Autodesk Inventor part; units mm, degrees
ref_plane "YZ Plane" through (0, 0, 0) normal (1, 0, 0) x (0, 1, 0)
ref_plane "XZ Plane" through (0, 0, 0) normal (0, 1, 0) x (-1, 0, 0)
ref_plane "XY Plane" through (0, 0, 0) normal (0, 0, 1) x (1, 0, 0)
sketch "Sketch1" plane through (0, 0, 0) normal (0, 0, 1) x (1, 0, 0)
  line L0 (0, 0) -> (609.6, 0)
  line L1 (609.6, 0) -> (609.6, 25.4)
  line L2 (609.6, 25.4) -> (0, 25.4)
  line L3 (0, 25.4) -> (0, 0)
  dimension "d0" = 25.4
  dimension "d1" = 609.6
extrude "Extrusion1" add sketch "Sketch1" along normal blind 25.4
shell "Shell1" thickness 1.5875 removed faces 2 at (0, 16.9333, 8.4667) at (609.6, 8.4667, 8.4667)
sketch "Sketch2" plane through (0, 0, 25.4) normal (0, 0, 1) x (1, 0, 0)
  line L0 (0, 0) -> (0, 25.4)
  line L1 (609.6, 25.4) -> (609.6, 0)
  line L2 (0, 25.4) -> (609.6, 25.4)
  line L3 (0, 1.5875) -> (0, 25.4)
  line L4 (25.4, 25.4) -> (0, 1.5875)
  line L5 (0, 25.4) -> (25.4, 25.4)
  line L6 (584.2, 25.4) -> (609.6, 25.4)
  line L7 (609.6, 25.4) -> (609.6, 1.5875)
  line L8 (609.6, 1.5875) -> (584.2, 25.4)
  dimension "d5" = 25.4
  dimension "d6" = 1.5875
  dimension "d7" = 25.4
  dimension "d8" = 1.5875
extrude "Extrusion2" cut sketch "Sketch2" against normal through all
sketch "Sketch3" plane through (0, 0, 0) normal (0, -1, 0) x (1, 0, 0)
  line L0 (0, 0) -> (0, 25.4)
  line L1 (0, 0) -> (609.6, 0)
  line L2 (609.6, 0) -> (609.6, 25.4)
  circle A0 centre (12.7, 12.7) radius 3.175
  circle A1 centre (596.9, 12.7) radius 3.175
  dimension "d11" = 12.7
  dimension "d12" = 12.7
  dimension "d13" = 6.35
  dimension "d14" = 12.7
  dimension "d15" = 12.7
extrude "Extrusion3" cut sketch "Sketch3" against normal through all
sketch "Sketch5" plane through (0, 0, 0) normal (0, -1, 0) x (1, 0, 0)
  circle A0 centre (12.7, 12.7) radius 3.175
  line L0 (0, 0) -> (0, 25.4)
  circle A1 centre (47.625, 12.7) radius 3.175
  circle A2 centre (149.225, 12.7) radius 3.175
  line L1 (12.7, 12.7) -> (47.625, 12.7) construction
  line L2 (47.625, 12.7) -> (149.225, 12.7) construction
  dimension "d23" = 6.35
  dimension "d25" = 47.625
  dimension "d26" = 101.6
extrude "Extrusion5" cut sketch "Sketch5" against normal through all contours A1 | A2
sketch "Sketch6" plane through (25.4, 25.4, 0) normal (0, 1, 0) x (1, 0, 0)
  circle A0 centre (123.825, -12.7) radius 3.175
  circle A1 centre (22.225, -12.7) radius 3.175
  circle A2 centre (22.225, -12.7) radius 6.35
  circle A3 centre (123.825, -12.7) radius 6.35
  point P0 (-25.4, 0)
  dimension "d29" = 12.7
  dimension "d30" = 12.7
extrude "Extrusion6" cut sketch "Sketch6" against normal up to next
properties material "Aluminum-6061"
The model under review builds one solid part; all positions refer to its coordinate system, in mm. A direction names the side the tool comes from. Give positions to 0.01 mm unless a question says otherwise; leave off trailing zeros. Loops run counter-clockwise (first coordinate to the right, second up) from the corner with the lowest first, then second, coordinate; pieces in that order, holes last. Notation, with made-up numbers: (32, -10.5) - (72, -10.5) arc R31 ccw to (72, 13.5) - close; hole circle Ø7 at (-7.75, 68.5). An arc over 180 degrees is marked (long way). Answer as a JSON object with one key per item and string values.
Q1. Insertion check: pin 1 (10 mm diameter, centred on x = 149.225, z = 12.7, fed in from +Y); pin 2 (10 mm diameter, centred on y = 9.5, z = 18.5, fed in from -X). Each pin has a flat end and moves straight along its axis. Give the tip position at first contact, or say it passes through.
Worked out:
{"pin 1": "stops at y = 1.59", "pin 2": "passes through"}
Q2. To check wall thickness, follow line 1 along Z through (x, y) = (379, 12.75); line 2 along Z through (x, y) = (596.9, 0.4) (3 decimals). State the ranges of each line that lie inside material, in increasing order.
Worked out:
{"line 1": "z = 0 to 1.59, 23.81 to 25.4", "line 2": "z = 0 to 9.525, 15.875 to 25.4"}
Q3. For faces 4 (the flat face through (309, 23.812, 13)), 5 (the cylindrical face through (155.28, 24.62, 10.79)), 6 (the flat face through (301, 13, 25.4)), list the 3-axis set-ups (+Z, -Z, +X, -X, +Y, -Y) from which the entire face can be reached by the end or side of a thin tool; tool diameter is ignored.
Worked out:
{"face 4": "+X, -X", "face 5": "+Y", "face 6": "+Z, +X, -X, +Y, -Y"}
Q4. Add section B-B on y = 16.75. State the section outline as (x, z) points, plus the area to 3 significant figures.
Worked out:
{"outline": "(16.17, 0) - (593.43, 0) - (593.43, 1.59) - (16.17, 1.59) - close; (16.17, 23.81) - (593.43, 23.81) - (593.43, 25.4) - (16.17, 25.4) - close", "area": "1,830 mm^2"}
Q5. Add section A-A on x = 112. State the section outline as (y, z) points.
Worked out:
{"outline": "(0, 0) - (25.4, 0) - (25.4, 25.4) - (0, 25.4) - close; hole (1.59, 1.59) - (23.81, 1.59) - (23.81, 23.81) - (1.59, 23.81) - close"}
Q6. Mouldability with a two-part tool opening along Y and no side actions: class faces 1 (the flat face through (301, 13, 1.588)), 2 (the flat face through (301, 13, 0)), 3 (the flat face through (301, 0, 13)) as +Y half, -Y half, draft (parallel to the pull), parting line (faces both ways), or undercut.
Worked out:
{"face 1": "undercut", "face 2": "draft", "face 3": "-Y half"}
